Autodesk Inventor part; units mm, degrees
ref_plane "YZ Plane" through (0, 0, 0) normal (1, 0, 0) x (0, 1, 0)
ref_plane "XZ Plane" through (0, 0, 0) normal (0, 1, 0) x (-1, 0, 0)
ref_plane "XY Plane" through (0, 0, 0) normal (0, 0, 1) x (1, 0, 0)
sketch "Sketch1" plane through (0, 0, 0) normal (0, 1, 0) x (-1, 0, 0)
  circle A0 centre (0, 0) radius 45.72
  dimension "d0" = 91.44
extrude "Extrusion1" add sketch "Sketch1" along normal blind 5.588
sketch "Sketch2" plane through (0, 5.588, 0) normal (0, 1, 0) x (1, 0, 0)
  circle A0 centre (0, 0) radius 38.1
  line L0 (0, 0) -> (-41.91, 0)
  line L1 (0, 0) -> (0, 41.91)
  line L2 (0, 0) -> (41.91, 0)
  line L3 (0, 0) -> (0, -41.91)
  circle A1 centre (-41.91, 0) radius 1.27
  circle A2 centre (0, -41.91) radius 1.27
  circle A3 centre (0, 41.91) radius 1.27
  circle A4 centre (41.91, 0) radius 1.27
  line L4 (0, 0) -> (0, -10.16)
  line L5 (0, -10.16) -> (-2.54, -10.16)
  line L6 (-2.54, -10.16) -> (2.54, -10.16)
  line L7 (2.54, -10.16) -> (2.54, 10.16)
  line L8 (2.54, 10.16) -> (-2.54, 10.16)
  line L9 (-2.54, 10.16) -> (-2.54, -10.16)
  line L10 (0, 0) -> (0, 15.24)
  circle A5 centre (0, 15.24) radius 1.016
  dimension "d3" = 76.2
  dimension "d4" = 41.91
  dimension "d5" = 41.91
  dimension "d6" = 41.91
  dimension "d7" = 41.91
  dimension "d8" = 2.54
  dimension "d9" = 2.54
  dimension "d10" = 2.54
  dimension "d11" = 2.54
  dimension "d12" = 10.16
  dimension "d13" = 2.54
  dimension "d14" = 5.08
  dimension "d15" = 20.32
  dimension "d16" = 15.24
  dimension "d17" = 2.032
extrude "Extrusion2" cut sketch "Sketch2" against normal blind 5.588 contours A2 | A1 | A3 | A4 | L7 L6 L3 L2 | L2 L1 L8 L7 | A5 L1 | L1 A5 | L5 L9 L0 L3 | L0 L9 L8 L1
properties part number "open1" material "Plastic, Transparent"
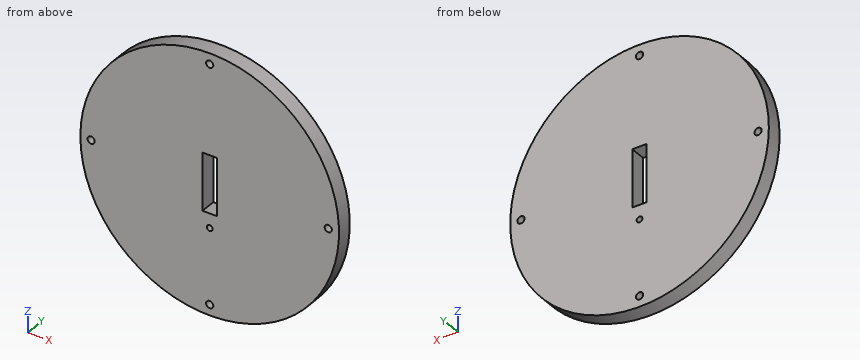
Design review of the part built by this model. Coordinates are the model's own, in mm. Round coordinates to 2 decimals unless told otherwise and drop trailing zeros. Write each loop counter-clockwise with the first axis right and the second up, starting at its lowest first coordinate (ties: lowest second). Pieces come first, ordered by that corner, then holes. Notation, with made-up numbers: (-2, -2.75) -> (54, -2.75) arc R23 cw to (54, 26.25) -> close; hole circle Ø8 at (77, -27.5). An arc over 180 degrees is marked (long way). Write item = value, one per line. Start each with the question number.
1) Take a section at C-C, the plane x = -41.91. State the section outline as (y, z) points, plus the area to 3 significant figures.
2) Clearance check with flat-ended pins moving along their axes: pin 1 (1.5 mm diameter, centred on x = -1, y = 4, fed in from +Z); pin 2 (3 mm diameter, centred on y = 3, z = 3.5, fed in from -X); pin 3 (3 mm diameter, centred on x = -4.5, y = 4.5, fed in from -Z). State where each tip first meets the part, or that it passes through.
3) Take a section at B-B, the plane y = 1.4. State the section outline as (x, z) points.
4) Wall thickness on probe 1 along Z at (x, y) = (0, 1.3); probe 2 along X at (y, z) = (2.5, -41.91); probe 3 along Z at (x, y) = (-41, 3): over which ranges is each line inside the solid? List them lowest first. Write a range as from..to.
5) Take a section at A-A, the plane z = 0. State the section outline as (x, y) points, plus the area to 3 significant figures.
6) Take a section at D-D, the plane z = 41.91. State the section outline as (x, y) points.
Results list:
q1.outline = (0, -18.27) -> (5.59, -18.27) -> (5.59, -1.27) -> (0, -1.27) -> close; (0, 1.27) -> (5.59, 1.27) -> (5.59, 18.27) -> (0, 18.27) -> close
q1.area = 190 mm²
q2.pin_1 = 45.72
q2.pin_2 = -45.68
q2.pin_3 = -45.62
q3.outline = circle Ø91.44 at (0, 0); hole circle Ø2.54 at (-41.91, 0); hole (-2.54, -10.16) -> (2.54, -10.16) -> (2.54, 10.16) -> (-2.54, 10.16) -> close; hole circle Ø2.54 at (0, -41.91); hole circle Ø2.54 at (0, 41.91); hole circle Ø2.03 at (0, -15.24); hole circle Ø2.54 at (41.91, 0)
q4.probe_1 = -45.72..-43.18, -40.64..-16.26, -14.22..-10.16, 10.16..40.64, 43.18..45.72
q4.probe_2 = -18.27..-1.27, 1.27..18.27
q4.probe_3 = -20.23..-0.89, 0.89..20.23
q5.outline = (-45.72, 0) -> (-43.18, 0) -> (-43.18, 5.59) -> (-45.72, 5.59) -> close; (-40.64, 0) -> (-2.54, 0) -> (-2.54, 5.59) -> (-40.64, 5.59) -> close; (2.54, 0) -> (40.64, 0) -> (40.64, 5.59) -> (2.54, 5.59) -> close; (43.18, 0) -> (45.72, 0) -> (45.72, 5.59) -> (43.18, 5.59) -> close
q5.area = 454 mm²
q6.outline = (-18.27, 0) -> (-1.27, 0) -> (-1.27, 5.59) -> (-18.27, 5.59) -> close; (1.27, 0) -> (18.27, 0) -> (18.27, 5.59) -> (1.27, 5.59) -> close
